Answer from the drawing. Dimensions are ordinates in mm from the lowest x, y and z of the part. A direction names the side the tool comes from. Coordinates: 2 decimals unless noted, no trailing zeros. Write each loop counter-clockwise with the first axis right and the second up, starting at its lowest first coordinate (ties: lowest second). Pieces come first, ordered by that corner, then holes. Notation, with made-up numbers: (37, 76) -> (73, 76) arc R20 ccw to (73, 80) -> close; hole circle Ø1 at (85, 89.25). An arc over 180 degrees is marked (long way). Return JSON: item names as keys, results as strings.
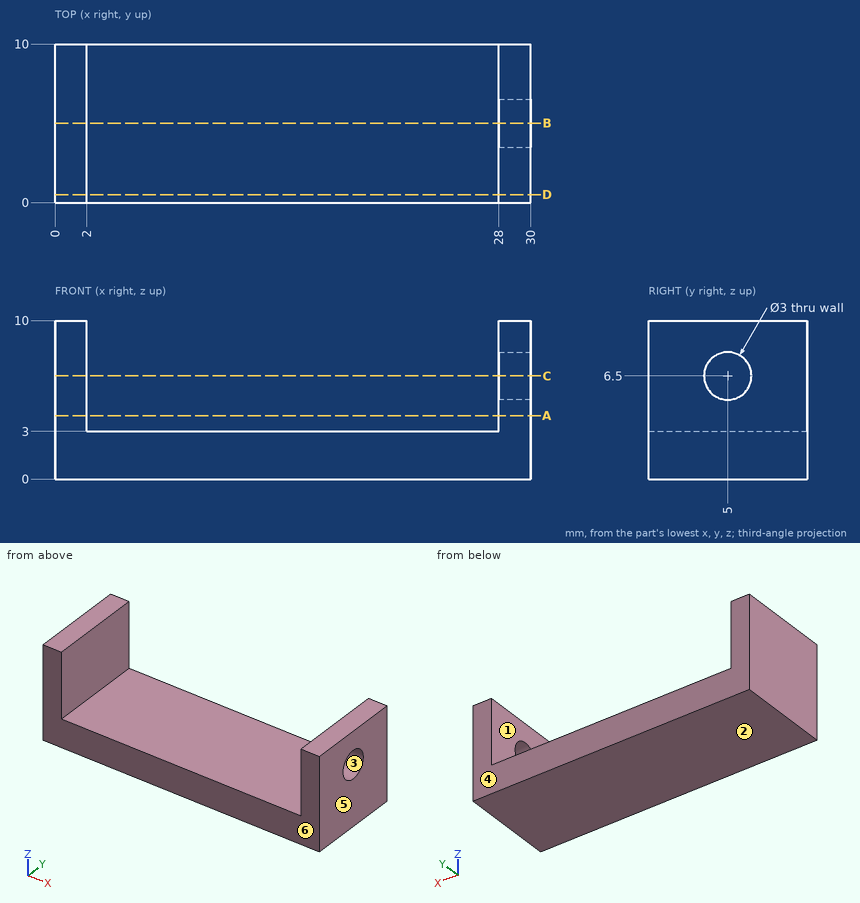
1. The part is cut by section D-D (y = 0.5). Determine the outline of the cut face in (x, z), then the cut area to 3 significant figures.
Taken from the geometry:
{"outline": "(0, 0) -> (30, 0) -> (30, 10) -> (28, 10) -> (28, 3) -> (2, 3) -> (2, 10) -> (0, 10) -> close", "area": "118 mm2"}
2. The part is cut by section A-A (z = 4). Determine the outline of the cut face in (x, y), then the cut area to 3 significant figures.
Taken from the geometry:
{"outline": "(0, 0) -> (2, 0) -> (2, 10) -> (0, 10) -> close; (28, 0) -> (30, 0) -> (30, 10) -> (28, 10) -> close", "area": "40.0 mm2"}
3. The part is cut by section B-B (y = 5). Determine the outline of the cut face in (x, z), then the cut area to 3 significant figures.
Taken from the geometry:
{"outline": "(0, 0) -> (30, 0) -> (30, 5) -> (28, 5) -> (28, 3) -> (2, 3) -> (2, 10) -> (0, 10) -> close; (28, 8) -> (30, 8) -> (30, 10) -> (28, 10) -> close", "area": "112 mm2"}
4. For a pull along Y with two mould halves and no side action, classify the marked faces 3, 4, 5 and 6 as +Y half, -Y half, draft (parallel to the pull), parting line (faces both ways), or undercut.
Taken from the geometry:
{"face 3": "undercut", "face 4": "+Y half", "face 5": "draft", "face 6": "-Y half"}
5. Consider L1, parallel to Y at x = 29.4, z = 6.5; L2, parallel to X at y = 9, z = 3.75; L3, parallel to Z at x = 15.75, y = 4.5. Determine where each line is inside the solid, lowest interval first.
Taken from the geometry:
{"L1": "y = 0 to 3.5, 6.5 to 10", "L2": "x = 0 to 2, 28 to 30", "L3": "z = 0 to 3"}
6. A tool of negligible diameter and unlimited length cuts with its end or side. For the marked faces 1 and 2, from which of +Z, -Z, +X, -X, +Y, -Y can it reach the whole face along a straight path? Write none if from no direction.
Taken from the geometry:
{"face 1": "+Z, +Y, -Y", "face 2": "-Z, +X, -X, +Y, -Y"}
7. The part is cut by section C-C (z = 6.5). Determine the outline of the cut face in (x, y), then the cut area to 3 significant figures.
Taken from the geometry:
{"outline": "(0, 0) -> (2, 0) -> (2, 10) -> (0, 10) -> close; (28, 0) -> (30, 0) -> (30, 3.5) -> (28, 3.5) -> close; (28, 6.5) -> (30, 6.5) -> (30, 10) -> (28, 10) -> close", "area": "34.0 mm2"}
